```python
from build123d import *

# Parameters (mm, degrees)
F0_W     = 22.5
F0_H     = 16
F0_H_2   = 2.5
F0_W_2   = 5
F0_H_3   = 4
F1_DEPTH = 11.7
F3_DEPTH = 4
F4_R     = 1.05
F5_DEPTH = 25
F6_R     = 2.375
F7_DEPTH = 3.5


with BuildPart() as f1:
    # F0 (on Front) → F1 (new body)
    with BuildSketch(Plane.XZ):
        with Locations((0, -3.25)):
            Rectangle(F0_W, F0_H)
        with Locations((0, 6)):
            Rectangle(F0_W, F0_H_2)
        with Locations((13.75, 6)):
            Rectangle(F0_W_2, F0_H_2)
        with Locations((-13.75, 6)):
            Rectangle(F0_W_2, F0_H_2)
        with Locations((0, 9.25)):
            Rectangle(F0_W, F0_H_3)
    extrude(amount=F1_DEPTH)

    # F2 (on face) → F3 (join)
    with BuildSketch(Plane.XY.offset(11.25)):
        with BuildLine():
            ThreePointArc((-0.1257874016, -3.3191540018), (-0.1800773211, -3.2089950347), (-0.2366677426, -3.1))
            ThreePointArc((-0.2366677426, -3.1), (-11.25, -5.85), (-0.2366677426, -8.6))
            ThreePointArc((-0.2366677426, -8.6), (-0.1800773211, -8.4910049653), (-0.1257874016, -8.3808459982))
            ThreePointArc((-0.1257874016, -8.3808459982), (-1.8, -5.85), (-0.1257874016, -3.3191540018))
        make_face()
        with BuildLine():
            Line((0.95, -3.1), (-0.2366677426, -3.1))
            ThreePointArc((-0.2366677426, -3.1), (-0.1800773211, -3.2089950347), (-0.1257874016, -3.3191540018))
            ThreePointArc((-0.1257874016, -3.3191540018), (0.4010585163, -3.1553454308), (0.95, -3.1))
        make_face()
        with BuildLine():
            ThreePointArc((-0.1257874016, -8.3808459982), (-0.1800773211, -8.4910049653), (-0.2366677426, -8.6))
            Line((-0.2366677426, -8.6), (0.95, -8.6))
            ThreePointArc((0.95, -8.6), (0.4010585163, -8.5446545692), (-0.1257874016, -8.3808459982))
        make_face()
        with BuildLine():
            ThreePointArc((0.95, -3.1), (0.4010585163, -3.1553454308), (-0.1257874016, -3.3191540018))
            ThreePointArc((-0.1257874016, -3.3191540018), (0.3042371839, -4.552241105), (0.45, -5.85))
            ThreePointArc((0.45, -5.85), (0.3042371839, -7.147758895), (-0.1257874016, -8.3808459982))
            ThreePointArc((-0.1257874016, -8.3808459982), (0.4010585163, -8.5446545692), (0.95, -8.6))
            ThreePointArc((0.95, -8.6), (2.8945436483, -7.7945436483), (3.7, -5.85))
            ThreePointArc((3.7, -5.85), (2.8945436483, -3.9054563517), (0.95, -3.1))
        make_face()
        with BuildLine():
            ThreePointArc((-0.1257874016, -8.3808459982), (0.3042371839, -7.147758895), (0.45, -5.85))
            ThreePointArc((0.45, -5.85), (0.3042371839, -4.552241105), (-0.1257874016, -3.3191540018))
            ThreePointArc((-0.1257874016, -3.3191540018), (-1.8, -5.85), (-0.1257874016, -8.3808459982))
        make_face()
    extrude(amount=F3_DEPTH)

    # F4 (on face) → F5 (cut)
    with BuildSketch(Plane.XY.offset(7.25)):
        with Locations((-13.75, -5.85)):
            Circle(F4_R)
        with Locations((13.75, -5.85)):
            Circle(F4_R)
    extrude(amount=-F5_DEPTH, mode=Mode.SUBTRACT)

    # F6 (on face) → F7 (join)
    with BuildSketch(Plane.XY.offset(15.25)):
        with Locations((-5.4, -5.85)):
            Circle(F6_R)
    extrude(amount=F7_DEPTH)


solid = f1.part
```
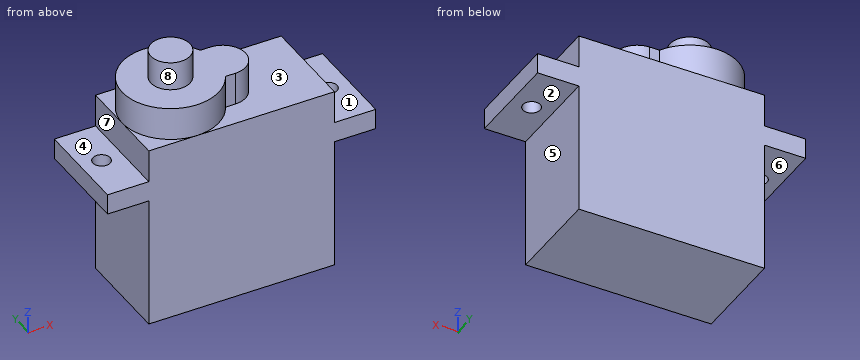
Can you work these out from the model? Positions are in its coordinate system, mm. Face numbers are marked on the shaded views. A direction names the side the tool comes from. Give positions to 0.01 mm unless a question says otherwise; leave off trailing zeros. Loops run counter-clockwise (first coordinate to the right, second up) from the corner with the lowest first, then second, coordinate; pieces in that order, holes last. Notation, with made-up numbers: M -14,64.5 L -9,64.5 A20 ccw -9,86.5 Z; hole C 28,40.25 d1. An arc over 180 degrees is marked long. One line per item, written item: value.
(1) We'd pull the mould along X, two halves only. Please class the marked faces 5, 6, 7 and 8: released by +X, released by -X, zero draft, split by the parting line, or undercut.
Returned:
face 5: released by +X
face 6: zero draft
face 7: released by -X
face 8: split by the parting line
(2) Which directions (+Z, -Z, +X, -X, +Y, -Y) give clear straight access to the entire face, cutting with the end or side of a thin tool? Please do the marked faces 1, 2, 3 and 4.
Returned:
face 1: +Z, +X, +Y, -Y
face 2: -Z, +X, +Y, -Y
face 3: +Z, +X
face 4: +Z, -X, +Y, -Y
(3) Suppose I cut it at A-A on x = -13.75. List the corners of the cut face in (y, z) for me.
Returned:
outline: M -11.7,4.75 L -6.9,4.75 L -6.9,7.25 L -11.7,7.25 Z; M -4.8,4.75 L 0,4.75 L 0,7.25 L -4.8,7.25 Z
(4) Suppose I cut it at D-D on y = -9.5. List the corners of the cut face in (x, z) for me, plus the area to 3 significant figures.
Returned:
outline: M -16.25,4.75 L -11.25,4.75 L -11.25,-11.25 L 11.25,-11.25 L 11.25,4.75 L 16.25,4.75 L 16.25,7.25 L 11.25,7.25 L 11.25,11.25 L -0.83,11.25 L -0.83,15.25 L -9.97,15.25 L -9.97,11.25 L -11.25,11.25 L -11.25,7.25 L -16.25,7.25 Z
area: 568 mm^2
(5) Suppose I cut it at C-C on x = -7. List the corners of the cut face in (y, z) for me.
Returned:
outline: M -11.7,-11.25 L 0,-11.25 L 0,11.25 L -0.22,11.25 L -0.22,15.25 L -4.09,15.25 L -4.09,18.75 L -7.61,18.75 L -7.61,15.25 L -11.48,15.25 L -11.48,11.25 L -11.7,11.25 Z
(6) I need wall thicknesses on line 1 (Y direction, x = 13.75, z = 6.55); line 2 (Z direction, x = 9, y = -7); line 3 (Z direction, x = -9, y = -6.25). Which ranges of each line are inside material? Lowest first, please.
Returned:
line 1: -11.7 to -6.9, -4.8 to 0
line 2: -11.25 to 11.25
line 3: -11.25 to 15.25
(7) Suppose I cut it at B-B on z = 13.75. List the corners of the cut face in (x, y) for me.
Returned:
outline: M -0.24,-8.6 L 0.95,-8.6 A2.75 ccw 0.95,-3.1 L -0.24,-3.1 A5.85 ccw long Z
(8) Will these pins go through, and if not, where does the flat tip stop? pin 1 (1.5 mm diameter, centred on x = 13.5, y = -3, fed in from +Z); pin 2 (1.2 mm diameter, centred on y = -7, z = 9, fed in from -X); pin 3 (3.5 mm diameter, centred on x = 2.5, y = -5.5, fed in from +Z).
Returned:
pin 1: z = 7.25
pin 2: x = -11.25
pin 3: z = 15.25
